Input: part model. Units: mm. Frame: model coordinates. A direction names the side the tool comes from. Coordinates: 2 decimals unless noted, no trailing zeros. Loops run counter-clockwise (first coordinate to the right, second up) from the corner with the lowest first, then second, coordinate; pieces in that order, holes last. Notation, with made-up numbers: (12.25, 39.25) - (39.25, 39.25) arc R18 cw to (39.25, 61.25) - close; hole circle Ø5 at (33.25, 27). An arc over 180 degrees is marked (long way). Use a Markdown table: item, result. Add a question column.
1. Access query for faces 1 (the face through (8, 0, 34)), 2 (the face through (5.305, 11.014, 36.535)), 3 (the face through (-0.195, -4.271, 1.513)). Directions: +Z, -Z, +X, -X, +Y, -Y. A direction counts if a zero-diameter tool reaches every point of the face in a straight line with its end or side. Return the directions, or none.
2. Contact query for flat-ended pins moving along their axis: P1, Ø1.8, axis at x = 5.5, y = 9.53, coming from the -Z side; P2, Ø4, axis at y = -5, z = 11.5, coming from the -X side (3 decimals); P3, Ø3.5, axis at x = 0, z = 10.5, coming from the +Y side (3 decimals); P4, Ø6, axis at x = -3, z = 27, coming from the -Y side (3 decimals). Output: stop coordinate, or through.
3. Ray query, L1, parallel to Z at x = 0, y = -3.6; L2, parallel to Y at x = 0, z = 7 (3 decimals); L3, parallel to Y at x = 0, z = 17 (3 decimals). Return the intervals inside material, ascending. Write a range as [from, to].
4. Draft query along Y for faces 4 (the face through (0.109, 2.976, 7.395)), 5 (the face through (16.692, 5.303, 35.479)), 6 (the face through (0, 0, 39)). Return one class per face: released by +Y, released by -Y, zero draft, split by the parting line, or undercut.
5. Section query B-B on z = 7. Return the cut outline in (x, y) (3 decimals).
6. Section query D-D on x = 5.5. State how many separate pieces and enclosed holes the cut face has, then the cut area to 3 significant figures.
7. Section query C-C on z = 31. Return the cut outline in (x, y) (3 decimals).
8. Section query A-A on x = 0. Return the cut outline in (y, z) (3 decimals).
```python
from build123d import *

# Parameters (mm, degrees)
ESQUISSE1_R             = 6.025
BOSS_EXTRU_1_DEPTH      = 34
ESQUISSE2_R             = 17.5
BOSS_EXTRU_2_DEPTH      = 5
ESQUISSE4_R             = 1.5
ENL_V_MAT_EXTRU_1_DEPTH = 10
CONG_1_R                = 2
ENL_V_MAT_EXTRU_2_DEPTH = 15
ESQUISSE6_R             = 1.5
ENL_V_MAT_EXTRU_3_DEPTH = 7


with BuildPart() as part:
    # Esquisse1 → Boss.-Extru.1 (new body)
    with BuildSketch(Plane.XY):
        Circle(ESQUISSE1_R)
    extrude(amount=BOSS_EXTRU_1_DEPTH)

    # Esquisse2 → Boss.-Extru.2 (add)
    with BuildSketch(Plane.XY.offset(34)):
        with Locations((0, 0.046797103)):
            Circle(ESQUISSE2_R)
    extrude(amount=BOSS_EXTRU_2_DEPTH)

    # Esquisse4 → Enlèv. mat.-Extru.1 (cut)
    with BuildSketch(Plane.XY.offset(39)):
        with Locations((-11, 0)):
            Circle(ESQUISSE4_R)
        with Locations((5.5, 9.526279442)):
            Circle(ESQUISSE4_R)
        with Locations((5.5, -9.526279442)):
            Circle(ESQUISSE4_R)
    extrude(amount=-ENL_V_MAT_EXTRU_1_DEPTH, mode=Mode.SUBTRACT)

    # Congé1
    cong_1_edges = [part.edges().sort_by_distance(p)[0] for p in [
        (-17.5, 0.046797103, 39),
    ]]
    fillet(cong_1_edges, radius=CONG_1_R)

    # Esquisse5 → Enlèv. mat.-Extru.2 (cut)
    with BuildSketch(Plane(origin=(0, 0, 0), x_dir=(-1, 0, 0), z_dir=(0, 0, -1))):
        with BuildLine():
            Line((1.525385197, -2.56), (-1.525385197, -2.56))
            ThreePointArc((-1.525385197, -2.56), (0, 2.978234065), (1.525385197, -2.56))
        make_face()
    extrude(amount=-ENL_V_MAT_EXTRU_2_DEPTH, mode=Mode.SUBTRACT)

    # Esquisse6 → Enlèv. mat.-Extru.3 (cut)
    with BuildSketch(Plane(origin=(0, 0, 0), x_dir=(1, 0, 0), z_dir=(0, 1, 0))):
        with Locations((0, -3)):
            Circle(ESQUISSE6_R)
    extrude(amount=-ENL_V_MAT_EXTRU_3_DEPTH, mode=Mode.SUBTRACT)


solid = part.part
```
Resolved:
| question | item | result |
|---|---|---|
| 1 | face 1 | -Z |
| 1 | face 2 | +Z, -Z |
| 1 | face 3 | -Y |
| 2 | P1 | through |
| 2 | P2 | x = -5.225 |
| 2 | P3 | y = 6.025 |
| 2 | P4 | y = -6.025 |
| 3 | L1 | [0, 1.5], [4.5, 39] |
| 3 | L2 | [-6.025, -2.56], [2.978, 6.025] |
| 3 | L3 | [-6.025, 6.025] |
| 4 | face 4 | undercut |
| 4 | face 5 | split by the parting line |
| 4 | face 6 | zero draft |
| 5 | outline | circle Ø12.05 at (0, 0); hole (-1.525, -2.56) - (1.525, -2.56) arc R2.979 ccw (long way) to start |
| 6 | separate pieces | 3 |
| 6 | enclosed holes | 0 |
| 6 | area | 302 mm² |
| 7 | outline | circle Ø12.05 at (0, 0) |
| 8 | outline | (-17.453, 34) - (-6.025, 34) - (-6.025, 4.5) - (-2.56, 4.5) - (-2.56, 15) - (2.978, 15) - (2.978, 0) - (6.025, 0) - (6.025, 34) - (17.547, 34) - (17.547, 37) arc R2 ccw to (15.547, 39) - (-15.453, 39) arc R2 ccw to (-17.453, 37) - close; (-6.025, 0) - (-2.56, 0) - (-2.56, 1.5) - (-6.025, 1.5) - close |
